The figure shows three views and two pictorial views of one solid part (mm, origin at its lowest corner). Answer the questions. Coordinates: 2 decimals unless noted, no trailing zeros. Loops run counter-clockwise (first coordinate to the right, second up) from the corner with the lowest first, then second, coordinate; pieces in that order, holes last. Notation, with made-up numbers: M 69.5,7.5 L 90.5,7.5 A15 cw 90.5,17.5 Z; hole C 37,48.25 d5. An arc over 180 degrees is marked long. One line per item, written item: value. Start each with the question number.
1. The part is cut by section A-A (z = 1.2). Write down the section's boundary in (x, y).
2. Flat-ended cylindrical pins translate along their axes: pin 1 (1 mm diameter, centred on x = 167, z = 1, fed in from +Y); pin 2 (1.3 mm diameter, centred on y = 79.5, z = 2, fed in from -X); pin 3 (1.6 mm diameter, centred on x = 326.5, z = 2, fed in from -Y). Find the tip coordinate at first contact, or state that the pin passes through.
3. The part is cut by section B-B (x = 127). Write down the section's boundary in (y, z) (3 decimals).
4. Consider probe 1 along Y at (x, z) = (330, 2.45); probe 2 along Y at (x, z) = (194, 1.5); probe 3 along X at (y, z) = (67.7, 2.3). Determine where each line is inside the solid, lowest interval first.
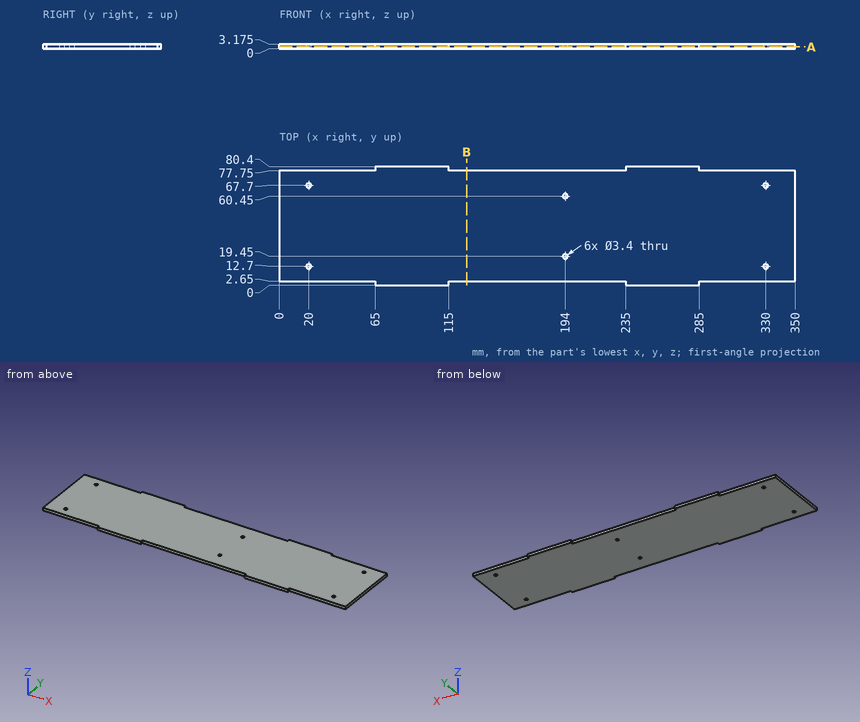
Answer block:
1. outline: M 0,2.65 L 65,2.65 L 65,0 L 115,0 L 115,2.65 L 235,2.65 L 235,0 L 285,0 L 285,2.65 L 350,2.65 L 350,77.75 L 285,77.75 L 285,80.4 L 235,80.4 L 235,77.75 L 115,77.75 L 115,80.4 L 65,80.4 L 65,77.75 L 0,77.75 Z; hole C 20,12.7 d3.4; hole C 20,67.7 d3.4; hole C 194,19.45 d3.4; hole C 194,60.45 d3.4; hole C 330,12.7 d3.4; hole C 330,67.7 d3.4
2. pin 1: stops at y = 77.75
2. pin 2: stops at x = 65
2. pin 3: stops at y = 2.65
3. outline: M 2.65,0 L 77.75,0 L 77.75,3.175 L 2.65,3.175 Z
4. probe 1: y = 2.65 to 11, 14.4 to 66, 69.4 to 77.75
4. probe 2: y = 2.65 to 17.75, 21.15 to 58.75, 62.15 to 77.75
4. probe 3: x = 0 to 18.3, 21.7 to 328.3, 331.7 to 350
